```python
from build123d import *

# Parameters (mm, degrees)
F1_DEPTH = 4
F0_W     = 5
F0_H     = 5
F2_DEPTH = 1


with BuildPart() as f1:
    # F0 (on Top) → F1 (new body)
    with BuildSketch(Plane.XY):
        Polygon((-2, 16), (-2, 11.5), (-7, 11.5), (-7, 2.5), (-2, 2.5), (-2, -2), (24.7, -2), (24.7, 2.5), (29.7, 2.5), (29.7, 11.5), (24.7, 11.5), (24.7, 16), align=None)
        Polygon((-6, 10.5), (-1, 10.5), (-1, 15), (23.7, 15), (23.7, 10.5), (28.7, 10.5), (28.7, 3.5), (23.7, 3.5), (23.7, -1), (-1, -1), (-1, 3.5), (-6, 3.5), align=None, mode=Mode.SUBTRACT)
    extrude(amount=F1_DEPTH)

    # F0 (on Top) → F2 (join)
    with BuildSketch(Plane.XY):
        Polygon((-1, 15), (-1, 10.5), (-6, 10.5), (-6, 3.5), (-1, 3.5), (-1, -1), (23.7, -1), (23.7, 3.5), (28.7, 3.5), (28.7, 10.5), (23.7, 10.5), (23.7, 15), align=None)
        Polygon((22.7, 0), (0, 0), (0, 4.5), (-5, 4.5), (-5, 9.5), (0, 9.5), (0, 14), (22.7, 14), (22.7, 9.5), (27.7, 9.5), (27.7, 4.5), (22.7, 4.5), align=None, mode=Mode.SUBTRACT)
        Polygon((0, 4.5), (0, 0), (22.7, 0), (22.7, 4.5), (22.7, 9.5), (22.7, 14), (0, 14), (0, 9.5), align=None)
        with Locations((-2.5, 7)):
            Rectangle(F0_W, F0_H)
        with Locations((25.2, 7)):
            Rectangle(F0_W, F0_H)
    extrude(amount=F2_DEPTH)


solid = f1.part
```
Design review of the part built by this model. Coordinates are the model's own, in mm. A direction names the side the tool comes from. Give positions to 0.01 mm unless a question says otherwise; leave off trailing zeros. Write each loop counter-clockwise with the first axis right and the second up, starting at its lowest first coordinate (ties: lowest second). Pieces come first, ordered by that corner, then holes.
(1) Add section D-D (z = 0.35). Give the boundary of the cut face in (x, y).
Checked values:
outline: (-7, 2.5) - (-2, 2.5) - (-2, -2) - (24.7, -2) - (24.7, 2.5) - (29.7, 2.5) - (29.7, 11.5) - (24.7, 11.5) - (24.7, 16) - (-2, 16) - (-2, 11.5) - (-7, 11.5) - close
(2) Wall thickness on line 1 along Y through (x, z) = (10.5, 3.15); line 2 along X through (y, z) = (1, 1.55); line 3 along Y through (x, z) = (24, 2.45): over which ranges is each line inside the solid? List them lowest first.
Checked values:
line 1: y = -2 to -1, 15 to 16
line 2: x = -2 to -1, 23.7 to 24.7
line 3: y = -2 to 3.5, 10.5 to 16
(3) Tool access review of faces 5 (the face through (11.3, 15.7, 4)), 6 (the face through (-2, 0, 2)), 7 (the face through (-7, 7, 2)), 8 (the face through (27, 11.5, 2)), 9 (the face through (23.7, 13, 2)): name each direction out of +Z, -Z, +X, -X, +Y, -Y from which nothing blocks a thin tool from reaching the whole face with its end or side.
Checked values:
face 5: +Z, +X, -X, +Y, -Y
face 6: +Z, -Z, -X, -Y
face 7: +Z, -Z, -X, +Y, -Y
face 8: +Z, -Z, +X, +Y
face 9: +Z
(4) Add section C-C (y = 0). Give the boundary of the cut face in (x, z).
Checked values:
outline: (-2, 0) - (24.7, 0) - (24.7, 4) - (23.7, 4) - (23.7, 1) - (-1, 1) - (-1, 4) - (-2, 4) - close
(5) Add section A-A (z = 3.15). Give the boundary of the cut face in (x, y), and give its area (3 significant figures).
Checked values:
outline: (-7, 2.5) - (-2, 2.5) - (-2, -2) - (24.7, -2) - (24.7, 2.5) - (29.7, 2.5) - (29.7, 11.5) - (24.7, 11.5) - (24.7, 16) - (-2, 16) - (-2, 11.5) - (-7, 11.5) - close; hole (-6, 3.5) - (-1, 3.5) - (-1, -1) - (23.7, -1) - (23.7, 3.5) - (28.7, 3.5) - (28.7, 10.5) - (23.7, 10.5) - (23.7, 15) - (-1, 15) - (-1, 10.5) - (-6, 10.5) - close
area: 105 mm2
(6) Mouldability with a two-part tool opening along X and no side actions: class faces 1 (the face through (-4, 11.5, 2)), 2 (the face through (23.7, 1, 2)), 3 (the face through (24.7, 0, 2)), 4 (the face through (-4, 10.5, 2)) as +X half, -X half, draft (parallel to the pull), parting line (faces both ways), or undercut.
Checked values:
face 1: draft
face 2: undercut
face 3: +X half
face 4: undercut
(7) Clearance check with flat-ended pins moving along their axes: pin 1 Ø1.5 at (y, z) = (1, 2) entering from +X; pin 2 Ø1.5 at (x, z) = (25, 1) entering from -Y; pin 3 Ø1.2 at (y, z) = (0.5, 2.5) entering from -X; pin 4 Ø0.9 at (x, z) = (25.5, 2.5) entering from -Y. State where each tip first meets the part, or that it passes through.
Checked values:
pin 1: stops at x = 24.7
pin 2: stops at y = -2
pin 3: stops at x = -2
pin 4: stops at y = 2.5
(8) Add section B-B (x = 12.5). Give the boundary of the cut face in (y, z), and give its area (3 significant figures).
Checked values:
outline: (-2, 0) - (16, 0) - (16, 4) - (15, 4) - (15, 1) - (-1, 1) - (-1, 4) - (-2, 4) - close
area: 24.0 mm2
